Here's how the part is built. I have some questions about the finished solid (model axes, mm). A direction names the side the tool comes from. Give positions to 0.01 mm unless a question says otherwise; leave off trailing zeros. Write each loop counter-clockwise with the first axis right and the second up, starting at its lowest first coordinate (ties: lowest second). Pieces come first, ordered by that corner, then holes. Notation, with made-up numbers: (3, 29) -> (30, 29) arc R25 cw to (30, 58) -> close; hole circle Ø11 at (-1, -15). An arc over 180 degrees is marked (long way). Use CSV: the item, a comma, the result in double quotes. Start each with the question number.
(1) For pin 1 Ø4.5 at (x, y) = (-48.5, 58.5) entering from +Z; pin 2 Ø2.5 at (x, y) = (-48.5, 58.5) entering from -Z, each with a flat end and sliding along its axis, tell me the tip position at first contact or that it passes through.
(2) Suppose I cut it at B-B on z = 12.5. List the corners of the cut face in (x, y) for me.
(3) Which directions (+Z, -Z, +X, -X, +Y, -Y) give clear straight access to the entire face, cutting with the end or side of a thin tool? Please do faces 4 (the cylindrical face through (23.934, -35.452, 0.74)), 5 (the flat face through (-13, 13, 6)), 6 (the flat face through (-54, 13, 16)).
(4) If we mould it in two halves opening along Y, with no side actions, what happens to faces 1 (the cylindrical face through (28, 64, 8)), 2 (the flat face through (-13, -37, 11)), 3 (the flat face through (-13, 13, 0))? For each: pulls with the +Y half, pulls with the -Y half, needs draft (parallel to the pull), parting line crosses it, or undercut.
(5) Suppose I cut it at C-C on x = -27.5. List the corners of the cut face in (y, z) for me.
(6) Suppose I cut it at A-A on y = -13.5. List the corners of the cut face in (x, z) for me, plus the area to 3 significant figures.
(7) I need wall thicknesses on L1, parallel to Y at x = -48.5, z = 4.8; L2, parallel to Y at x = -44.5, z = 11.5; L3, parallel to X at y = -29.5, z = 10.5. Which ranges of each line are inside material? Lowest first, please. Write a range as [from, to].
from build123d import *

# Parameters (mm, degrees)
SKETCH1_W           = 85
SKETCH1_H           = 105
BOSS_EXTRUDE1_DEPTH = 16
SKETCH2_W           = 79
SKETCH2_H           = 99
CUT_EXTRUDE1_DEPTH  = 10
FILLET1_R           = 5
SKETCH3_R           = 2
CUT_EXTRUDE2_DEPTH  = 1.5
SKETCH4_R           = 1.35
CUT_EXTRUDE3_DEPTH  = 87.372738755
FILLET2_R           = 3


with BuildPart() as part:
    # Sketch1 → Boss-Extrude1 (new body)
    with BuildSketch(Plane.XY):
        with Locations((-12.5, 12.5)):
            Rectangle(SKETCH1_W, SKETCH1_H)
    extrude(amount=BOSS_EXTRUDE1_DEPTH)

    # Sketch2 → Cut-Extrude1 (cut)
    with BuildSketch(Plane.XY.offset(16)):
        with Locations((-12.5, 12.5)):
            Rectangle(SKETCH2_W, SKETCH2_H)
    extrude(amount=-CUT_EXTRUDE1_DEPTH, mode=Mode.SUBTRACT)

    # Fillet1
    fillet1_edges = [part.edges().sort_by_distance(p)[0] for p in [
        (-55, 65, 8),
        (30, 65, 8),
        (30, -40, 8),
        (-55, -40, 8),
    ]]
    fillet(fillet1_edges, radius=FILLET1_R)

    # Sketch3 → Cut-Extrude2 (cut)
    with BuildSketch(Plane(origin=(0, 0, 0), x_dir=(-1, 0, 0), z_dir=(0, 0, -1))):
        with Locations((48.5, 58.5)):
            Circle(SKETCH3_R)
        with Locations((-23.5, -33.5)):
            Circle(SKETCH3_R)
    extrude(amount=-CUT_EXTRUDE2_DEPTH, mode=Mode.SUBTRACT)

    # Sketch4 → Cut-Extrude3 (cut, through all)
    with BuildSketch(Plane(origin=(0, 0, 1.5), x_dir=(-1, 0, 0), z_dir=(0, 0, -1))):
        with Locations((48.5, 58.5)):
            Circle(SKETCH4_R)
        with Locations((-23.5, -33.5)):
            Circle(SKETCH4_R)
    extrude(amount=-CUT_EXTRUDE3_DEPTH, mode=Mode.SUBTRACT)

    # Fillet2
    fillet2_edges = [part.edges().sort_by_distance(p)[0] for p in [
        (-52, -37, 11),
        (-52, 62, 11),
        (27, 62, 11),
        (27, -37, 11),
    ]]
    fillet(fillet2_edges, radius=FILLET2_R)


solid = part.part
Geometry says:
1,pin 1,"z = 6"
1,pin 2,"through"
2,outline,"(-55, -35) arc R5 ccw to (-50, -40) -> (25, -40) arc R5 ccw to (30, -35) -> (30, 60) arc R5 ccw to (25, 65) -> (-50, 65) arc R5 ccw to (-55, 60) -> close; hole (-52, -34) arc R3 ccw to (-49, -37) -> (24, -37) arc R3 ccw to (27, -34) -> (27, 59) arc R3 ccw to (24, 62) -> (-49, 62) arc R3 ccw to (-52, 59) -> close"
3,face 4,"-Z"
3,face 5,"+Z"
3,face 6,"+Z, +X, -X, +Y, -Y"
4,face 1,"pulls with the +Y half"
4,face 2,"undercut"
4,face 3,"needs draft"
5,outline,"(-40, 0) -> (65, 0) -> (65, 16) -> (62, 16) -> (62, 6) -> (-37, 6) -> (-37, 16) -> (-40, 16) -> close"
6,outline,"(-55, 0) -> (30, 0) -> (30, 16) -> (27, 16) -> (27, 6) -> (-52, 6) -> (-52, 16) -> (-55, 16) -> close"
6,area,"570 mm²"
7,L1,"[-40, 57.15], [59.85, 65]"
7,L2,"[-40, -37], [62, 65]"
7,L3,"[-55, -52], [27, 30]"
